```python
from build123d import *

# Parameters (mm, degrees)
F0_W     = 254
F0_H     = 50.8
F0_R     = 3.175
F0_R_2   = 6
F1_DEPTH = 10
F2_R     = 11
F2_R_2   = 6
F3_DEPTH = 7
F4_R     = 3.175
F5_DEPTH = 5.08


with BuildPart() as f1:
    # F0 (on Top) → F1 (new body)
    with BuildSketch(Plane.XY):
        Rectangle(F0_W, F0_H)
        with Locations((-114.3, -12.7)):
            Circle(F0_R, mode=Mode.SUBTRACT)
        with Locations((-25.4, 0)):
            Circle(F0_R_2, mode=Mode.SUBTRACT)
        with Locations((114.3, -12.7)):
            Circle(F0_R, mode=Mode.SUBTRACT)
        with Locations((25.4, 0)):
            Circle(F0_R_2, mode=Mode.SUBTRACT)
        with Locations((-114.3, 12.7)):
            Circle(F0_R, mode=Mode.SUBTRACT)
        with Locations((114.3, 12.7)):
            Circle(F0_R, mode=Mode.SUBTRACT)
    extrude(amount=F1_DEPTH)

    # F2 (on face) → F3 (cut)
    with BuildSketch(Plane.XY.offset(10)):
        with Locations((-25.4, 0)):
            Circle(F2_R)
        with Locations((-25.4, 0)):
            Circle(F2_R_2, mode=Mode.SUBTRACT)
        with Locations((25.4, 0)):
            Circle(F2_R)
        with Locations((25.4, 0)):
            Circle(F2_R_2, mode=Mode.SUBTRACT)
    extrude(amount=-F3_DEPTH, mode=Mode.SUBTRACT)

    # F4 (on face) → F5 (cut)
    with BuildSketch(Plane(origin=(0, 0, 0), x_dir=(1, 0, 0), z_dir=(0, 0, -1))):
        Polygon((-111.000443, 18.415), (-117.599557, 18.415), (-120.899114, 12.7), (-117.599557, 6.985), (-111.000443, 6.985), (-107.700886, 12.7), align=None)
        with Locations((-114.3, 12.7)):
            Circle(F4_R, mode=Mode.SUBTRACT)
        Polygon((-111.000443, -6.985), (-117.599557, -6.985), (-120.899114, -12.7), (-117.599557, -18.415), (-111.000443, -18.415), (-107.700886, -12.7), align=None)
        with Locations((-114.3, -12.7)):
            Circle(F4_R, mode=Mode.SUBTRACT)
        Polygon((117.599557, -6.985), (111.000443, -6.985), (107.700886, -12.7), (111.000443, -18.415), (117.599557, -18.415), (120.899114, -12.7), align=None)
        with Locations((114.3, -12.7)):
            Circle(F4_R, mode=Mode.SUBTRACT)
        Polygon((117.599557, 18.415), (111.000443, 18.415), (107.700886, 12.7), (111.000443, 6.985), (117.599557, 6.985), (120.899114, 12.7), align=None)
        with Locations((114.3, 12.7)):
            Circle(F4_R, mode=Mode.SUBTRACT)
    extrude(amount=-F5_DEPTH, mode=Mode.SUBTRACT)


solid = f1.part
```
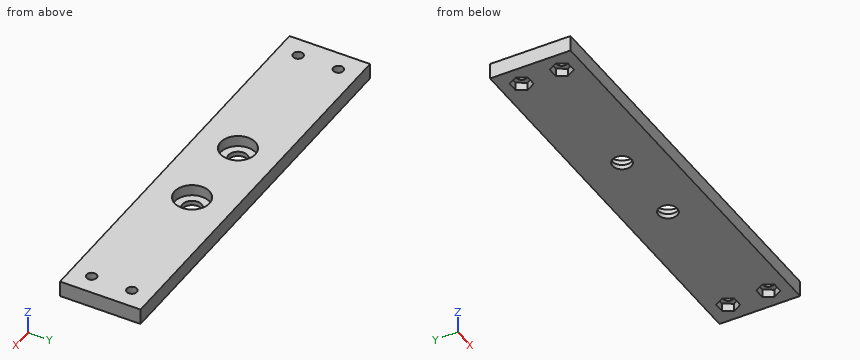
Geometry: final body of the model. Coordinates: model frame, mm. Round coordinates to 2 decimals unless told otherwise and drop trailing zeros. Order: outer loops, then holes, each group sorted by start corner. A loop starts at its lowest first (then second) coordinate and runs counter-clockwise, first axis right, second up. Notation, with made-up numbers: (5.5, -7) -> (36.5, -7) arc R18 cw to (36.5, -3) -> close; hole circle Ø2 at (37, 48.5). An arc over 180 degrees is marked (long way). Use CSV: the item, a comma, the result in double quotes. Start each with the question number.
1) Material intervals for line 1 along X through (y, z) = (-12.7, 8.9) (3 decimals); line 2 along Y through (x, z) = (114.3, 8.35) (3 decimals); line 3 along Y through (x, z) = (25.4, 2.45), sorted ascending. Write a range as from..to.
2) Section B-B (z = 7.5). Return the cut outline in (x, y) (3 decimals).
3) Section A-A (x = -25.4). Return the cut outline in (y, z).
4) First-contact query: pin 1 Ø1 at (x, y) = (-42.5, -2) entering from -Z; pin 2 Ø5.5 at (x, y) = (114.3, 12.7) entering from +Z; pin 3 Ø5.5 at (x, y) = (112, -12) entering from -Z; pin 4 Ø19 at (x, y) = (-25.4, 0) entering from +Z. Flat tips, straight axial feed; report the tip coordinate or a pass-through.
Returned:
1,line 1,"x = -127..-117.475, -111.125..111.125, 117.475..127"
1,line 2,"y = -25.4..-15.875, -9.525..9.525, 15.875..25.4"
1,line 3,"y = -25.4..-6, 6..25.4"
2,outline,"(-127, -25.4) -> (127, -25.4) -> (127, 25.4) -> (-127, 25.4) -> close; hole circle Ø6.35 at (-114.3, -12.7); hole circle Ø6.35 at (-114.3, 12.7); hole circle Ø22 at (-25.4, 0); hole circle Ø22 at (25.4, 0); hole circle Ø6.35 at (114.3, -12.7); hole circle Ø6.35 at (114.3, 12.7)"
3,outline,"(-25.4, 0) -> (-6, 0) -> (-6, 3) -> (-11, 3) -> (-11, 10) -> (-25.4, 10) -> close; (6, 0) -> (25.4, 0) -> (25.4, 10) -> (11, 10) -> (11, 3) -> (6, 3) -> close"
4,pin 1,"stops at z = 0"
4,pin 2,"passes through"
4,pin 3,"stops at z = 5.08"
4,pin 4,"stops at z = 3"
